Source: CAD feature listing. Evaluate the final solid. Frame: model axes, mm. Face numbers are marked on the shaded views. Coordinates: 2 decimals unless noted, no trailing zeros. Loops run counter-clockwise (first coordinate to the right, second up) from the corner with the lowest first, then second, coordinate; pieces in that order, holes last.
```python
from build123d import *

# Parameters (mm, degrees)
SKETCH1_R                    = 3.175
SKETCH1_R_2                  = 1.5875
BOSS_EXTRUDE1_DEPTH          = 6.35
F_10_0_1935_DIAMETER_HOLE1_D = 4.9149


with BuildPart() as part:
    # Sketch1 → Boss-Extrude1 (new body)
    with BuildSketch(Plane(origin=(0, 0, 0), x_dir=(1, 0, 0), z_dir=(0, 1, 0))):
        with BuildLine():
            Line((-20.32, 21.59), (-15.875, 21.59))
            Line((-15.875, 21.59), (-15.875, 27.94))
            Line((-15.875, 27.94), (15.875, 27.94))
            Line((15.875, 27.94), (15.875, 21.59))
            Line((15.875, 21.59), (20.32, 21.59))
            ThreePointArc((20.32, 21.59), (41.91, 0), (20.32, -21.59))
            Line((20.32, -21.59), (20.32, -31.115))
            Line((20.32, -31.115), (-20.32, -31.115))
            Line((-20.32, -31.115), (-20.32, -21.59))
            ThreePointArc((-20.32, -21.59), (-41.91, 0), (-20.32, 21.59))
        make_face()
        with Locations(Location((20.32, 0, 0), (0, 0, 270))):
            Circle(SKETCH1_R, mode=Mode.SUBTRACT)
        with Locations(Location((7.62, 21.997045256, 0), (0, 0, 270))):
            Circle(SKETCH1_R_2, mode=Mode.SUBTRACT)
        with Locations(Location((-20.32, 0, 0), (0, 0, 270))):
            Circle(SKETCH1_R, mode=Mode.SUBTRACT)
        with Locations(Location((-7.62, 21.997045256, 0), (0, 0, 270))):
            Circle(SKETCH1_R_2, mode=Mode.SUBTRACT)
    extrude(amount=BOSS_EXTRUDE1_DEPTH)

    # #10 (0.1935) Diameter Hole1 (through all)
    with Locations(Plane(origin=(0, 6.35, 0), x_dir=(1, 0, 0), z_dir=(0, 1, 0))):
        with Locations((0, 21.997045256), (-7.62, -24.765), (7.62, -24.765)):
            Hole(F_10_0_1935_DIAMETER_HOLE1_D / 2)


solid = part.part
```
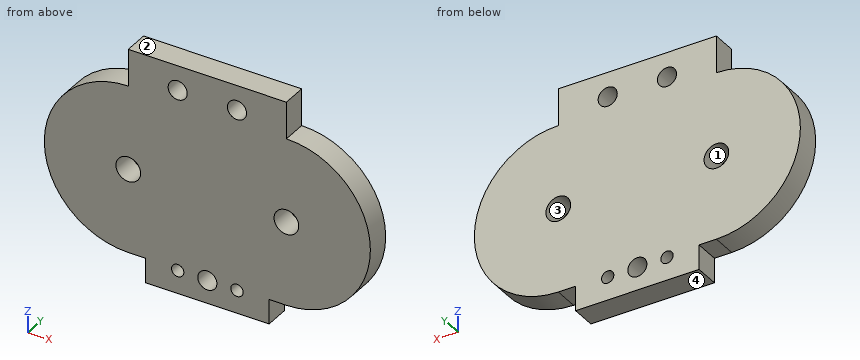
Q1. Section query A-A on z = 0. Return the cut outline in (x, y) (3 decimals).
Q2. Section query D-D on y = 4.5. Count the separate pieces of the cut face and the enclosed holes in it, then the cut area to 3 significant figures.
Q3. Section query C-C on x = -22. Return the cut outline in (y, z).
Q4. Material intervals for line 1 along Z through (x, y) = (20, 5.25) (3 decimals); line 2 along X through (y, z) = (5, 1.5); line 3 along X through (y, z) = (3, -17), sorted ascending.
Q5. First-contact query: pin 1 Ø4.5 at (x, z) = (7.62, 24.765) entering from -Y; pin 2 Ø1.9 at (y, z) = (2, -25) entering from +X (3 decimals); pin 3 Ø1.5 at (y, z) = (5, 2) entering from -X; pin 4 Ø1.3 at (x, y) = (19, 4.5) entering from -Z. Flat tips, straight axial feed; report the tip coordinate or a pass-through.
Q6. Draft query along Z for the marked faces 1, 2, 3 and 4. Return one class per face: released by +Z, released by -Z, zero draft, split by the parting line, or undercut.
Q7. Section query B-B on x = -7.62. Return the cut outline in (y, z) (3 decimals), then the cut area to 3 significant figures.
Resolved:
1. outline: (-41.91, 0) - (-23.495, 0) - (-23.495, 6.35) - (-41.91, 6.35) - close; (-17.145, 0) - (17.145, 0) - (17.145, 6.35) - (-17.145, 6.35) - close; (23.495, 0) - (41.91, 0) - (41.91, 6.35) - (23.495, 6.35) - close
2. separate pieces: 1
2. enclosed holes: 7
2. area: 3,670 mm2
3. outline: (0, -21.52) - (6.35, -21.52) - (6.35, -2.69) - (0, -2.69) - close; (0, 2.69) - (6.35, 2.69) - (6.35, 21.52) - (0, 21.52) - close
4. line 1: z = -21.59 to -3.159, 3.159 to 31.115
4. line 2: x = -41.86 to -23.12, -17.52 to 17.52, 23.12 to 41.86
4. line 3: x = -33.63 to 33.63
5. pin 1: passes through
5. pin 2: stops at x = 15.875
5. pin 3: stops at x = -41.87
5. pin 4: stops at z = -21.59
6. face 1: undercut
6. face 2: released by +Z
6. face 3: undercut
6. face 4: released by -Z
7. outline: (0, -27.94) - (6.35, -27.94) - (6.35, -23.585) - (0, -23.585) - close; (0, -20.41) - (6.35, -20.41) - (6.35, 22.308) - (0, 22.308) - close; (0, 27.222) - (6.35, 27.222) - (6.35, 31.115) - (0, 31.115) - close
7. area: 324 mm2
